For this review, take the finished solid that the model builds, in its own axes (mm). A direction names the side the tool comes from. Give positions to 0.01 mm unless a question says otherwise; leave off trailing zeros. Order: outer loops, then holes, each group sorted by start corner. A loop starts at its lowest first (then second) coordinate and runs counter-clockwise, first axis right, second up. Notation, with made-up numbers: (7, -16.5) - (24, -16.5) arc R20 ccw to (24, 2.5) - close; hole circle Ø10 at (-9, -4). An arc over 180 degrees is marked (long way). Use a Markdown table: item, result. Add a question column.
1) Clearance check with flat-ended pins moving along their axes: P1, Ø1.5, axis at y = 39.5, z = -7, coming from the +X side; P2, Ø17, axis at x = 5.5, z = -1, coming from the -Y side; P3, Ø3.5, axis at y = 20, z = 0, coming from the -X side; P4, Ø5, axis at x = 36.5, z = -13.5, coming from the +Y side. State where each tip first meets the part, or that it passes through.
2) Mouldability with a two-part tool opening along X and no side actions: class faces 4 (the face through (3, 0, -3)), 5 (the face through (5.072, -15.107, 15.965)), 6 (the face through (16, -10, 16)) as released by +X, released by -X, zero draft, split by the parting line, or undercut.
3) We need section A-A on y = 40. Write out the cut boundary in (x, z).
4) Machinability: for faces 1 (the face through (25, 34, 4)), 2 (the face through (33, 8, -12)), 3 (the face through (7, -6, 13.5)), which of the approach directions +Z, -Z, +X, -X, +Y, -Y give a long, thin tool a straight path to every point of the face, cutting with its end or side? Answer none if there is none.
5) We need section C-C on x = 17.5. Write out the cut boundary in (y, z), then the cut area to 3 significant figures.
6) Wall thickness on L1, parallel to Y at x = -16, z = 0; L2, parallel to Z at x = 21, y = 20; L3, parallel to X at y = 34.5, z = -16.5: over which ranges is each line inside the solid? List them lowest first.
7) We need section D-D on z = 0. Write out the cut boundary in (x, y), then the cut area to 3 significant figures.
```python
from build123d import *

# Parameters (mm, degrees)
SKETCH_1_W             = 45
SKETCH_1_H             = 38.5
EXTRUDE_1_DEPTH        = 60
SKETCH_2_R             = 15.1
CUT_EXTRUDE_1_DEPTH    = 50
SKETCH_3_R             = 2.5
EXTRUDE_2_DEPTH        = 5
SKETCH_4_R             = 1.5
CUT_EXTRUDE_2_DEPTH    = 78.620873481
PATTERN_LINEAR_1_COUNT = 2
PATTERN_LINEAR_1_PITCH = 20
FILLET_1_R             = 10
SKETCH_5_R             = 4
EXTRUDE_3_DEPTH        = 8
FILLET_2_R             = 15


with BuildPart() as part:
    # 草圖1 → 填料-伸長1 (new body)
    with BuildSketch(Plane(origin=(0, 0, 0), x_dir=(1, 0, 0), z_dir=(0, 1, 0))):
        with Locations((2.5, 0.75)):
            Rectangle(SKETCH_1_W, SKETCH_1_H)
    extrude(amount=EXTRUDE_1_DEPTH)

    # 草圖2 → 除料-伸長1 (cut)
    with BuildSketch(Plane(origin=(0, 60, 0), x_dir=(1, 0, 0), z_dir=(0, 1, 0))):
        with Locations(Location((0, 0, 0), (0, 0, 270))):
            Circle(SKETCH_2_R)
    extrude(amount=-CUT_EXTRUDE_1_DEPTH, mode=Mode.SUBTRACT)

    # 草圖3 → 填料-伸長2 (add)
    with BuildSketch(Plane.XY.offset(18.5)):
        Polygon((-20, 0), (5, -15.5), (25, -15.5), (25, 0), align=None)
        with Locations((17.5, -8)):
            Circle(SKETCH_3_R, mode=Mode.SUBTRACT)
    extrude(amount=-EXTRUDE_2_DEPTH)

    # 草圖4 → 除料-伸長2 (cut, through all)
    with BuildSketch(Plane(origin=(25, 0, 0), x_dir=(0, 0, -1), z_dir=(1, 0, 0))):
        with Locations((0, 20)):
            Circle(SKETCH_4_R)
    cut_extrude_2 = extrude(amount=-CUT_EXTRUDE_2_DEPTH, mode=Mode.SUBTRACT)

    # 直線複製排列1: 除料-伸長2 ×2
    with Locations(*[(0, i * PATTERN_LINEAR_1_PITCH, 0) for i in range(1, PATTERN_LINEAR_1_COUNT)]):
        add(cut_extrude_2, mode=Mode.SUBTRACT)

    # 圓角1
    fillet_1_edges = [part.edges().sort_by_distance(p)[0] for p in [
        (25, -15.5, 16),
        (5, -15.5, 16),
    ]]
    fillet(fillet_1_edges, radius=FILLET_1_R)

    # 草圖5 → 填料-伸長3 (add)
    with BuildSketch(Plane(origin=(0, 0, -20), x_dir=(-1, 0, 0), z_dir=(0, 0, -1))):
        with BuildLine():
            Line((-25, 0), (-40, 0))
            ThreePointArc((-40, 0), (-47, 7), (-40, 14))
            Line((-40, 14), (-25, 14))
            Line((-25, 14), (-25, 0))
        make_face()
        with Locations((-40, 7)):
            Circle(SKETCH_5_R, mode=Mode.SUBTRACT)
    extrude(amount=-EXTRUDE_3_DEPTH)

    # 圓角2
    fillet_2_edges = [part.edges().sort_by_distance(p)[0] for p in [
        (25, 14, -16),
    ]]
    fillet(fillet_2_edges, radius=FILLET_2_R - 0.0001)  # a hair under: the kernel refuses the full size


solid = part.part
```
Checked values:
| question | item | result |
|---|---|---|
| 1 | P1 | x = 25 |
| 1 | P2 | y = 0 |
| 1 | P3 | x = -20 |
| 1 | P4 | y = 15.25 |
| 2 | face 4 | zero draft |
| 2 | face 5 | released by -X |
| 2 | face 6 | undercut |
| 3 | outline | (-20, -20) - (25, -20) - (25, -1.5) - (15.03, -1.5) arc R15.1 cw to (-15.03, -1.5) - (-20, -1.5) - close; (-20, 1.5) - (-15.03, 1.5) arc R15.1 cw to (15.03, 1.5) - (25, 1.5) - (25, 18.5) - (-20, 18.5) - close |
| 4 | face 1 | +Z, +X, +Y |
| 4 | face 2 | +Z, +X, +Y, -Y |
| 4 | face 3 | -Z, +X, -X, -Y |
| 5 | outline | (-15.18, 13.5) - (-10.5, 13.5) - (-10.5, 18.5) - (-15.18, 18.5) - close; (-5.5, 13.5) - (0, 13.5) - (0, -20) - (60, -20) - (60, 18.5) - (-5.5, 18.5) - close; hole circle Ø3 at (20, 0); hole circle Ø3 at (40, 0) |
| 5 | area | 2,350 mm² |
| 6 | L1 | 0 to 18.5, 21.5 to 38.5, 41.5 to 60 |
| 6 | L2 | -20 to -1.5, 1.5 to 18.5 |
| 6 | L3 | -20 to 25 |
| 7 | outline | (-20, 0) - (25, 0) - (25, 18.5) - (15.1, 18.5) - (15.1, 10) - (-15.1, 10) - (-15.1, 18.5) - (-20, 18.5) - close; (-20, 21.5) - (-15.1, 21.5) - (-15.1, 38.5) - (-20, 38.5) - close; (-20, 41.5) - (-15.1, 41.5) - (-15.1, 60) - (-20, 60) - close; (15.1, 21.5) - (25, 21.5) - (25, 38.5) - (15.1, 38.5) - close; (15.1, 41.5) - (25, 41.5) - (25, 60) - (15.1, 60) - close |
| 7 | area | 1,100 mm² |
